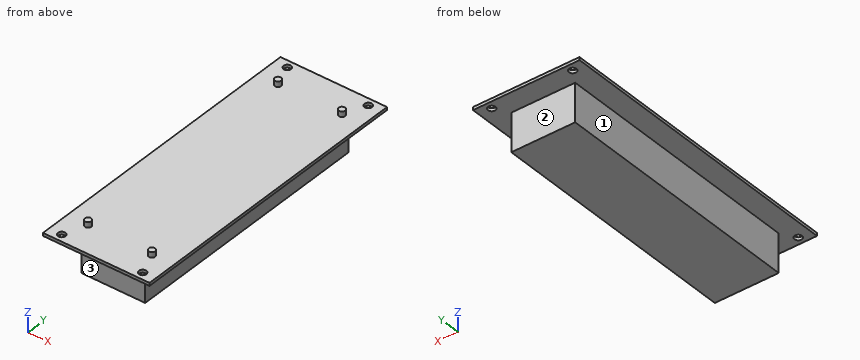
from build123d import *

# Parameters (mm, degrees)
SKETCH1_W           = 50
SKETCH1_H           = 140
BOSS_EXTRUDE1_DEPTH = 0.7
SKETCH3_W           = 30
SKETCH3_H           = 120
BOSS_EXTRUDE2_DEPTH = 18
SKETCH4_R           = 1.75
CUT_EXTRUDE1_DEPTH  = 1.4
SKETCH5_R           = 1.5
BOSS_EXTRUDE3_DEPTH = 2.5


with BuildPart() as part:
    # Sketch1 → Boss-Extrude1 (new, symmetric)
    with BuildSketch(Plane.XY):
        Rectangle(SKETCH1_W, SKETCH1_H)
    extrude(amount=BOSS_EXTRUDE1_DEPTH, both=True)

    # Sketch3 → Boss-Extrude2 (add)
    with BuildSketch(Plane(origin=(0, 0, -0.7), x_dir=(-1, 0, 0), z_dir=(0, 0, -1))):
        Rectangle(SKETCH3_W, SKETCH3_H)
    extrude(amount=BOSS_EXTRUDE2_DEPTH)

    # Sketch4 → Cut-Extrude1 (cut)
    with BuildSketch(Plane(origin=(0, 0, -0.7), x_dir=(-1, 0, 0), z_dir=(0, 0, -1))):
        with Locations((-19, 66.5)):
            Circle(SKETCH4_R)
        with Locations((19, 66.5)):
            Circle(SKETCH4_R)
        with Locations((-19, -66.5)):
            Circle(SKETCH4_R)
        with Locations((19, -66.5)):
            Circle(SKETCH4_R)
    extrude(amount=-CUT_EXTRUDE1_DEPTH, mode=Mode.SUBTRACT)

    # Sketch5 → Boss-Extrude3 (add)
    with BuildSketch(Plane.XY.offset(0.7)):
        with Locations(Location((15, 56, 0), (0, 0, 180))):
            Circle(SKETCH5_R)
        with Locations(Location((-15, 56, 0), (0, 0, 180))):
            Circle(SKETCH5_R)
        with Locations(Location((-15, -56, 0), (0, 0, 180))):
            Circle(SKETCH5_R)
        with Locations(Location((15, -56, 0), (0, 0, 180))):
            Circle(SKETCH5_R)
    extrude(amount=BOSS_EXTRUDE3_DEPTH)


solid = part.part
Source: CAD feature listing. Evaluate the final solid. Frame: model axes, mm. Face numbers are marked on the shaded views. A direction names the side the tool comes from. Round coordinates to 2 decimals unless told otherwise and drop trailing zeros. Loops run counter-clockwise (first coordinate to the right, second up) from the corner with the lowest first, then second, coordinate; pieces in that order, holes last.
Q1. Access query for the marked faces 1, 2 and 3. Directions: +Z, -Z, +X, -X, +Y, -Y. A direction counts if a zero-diameter tool reaches every point of the face in a straight line with its end or side. Return the directions, or none.
Q2. First-contact query: P1, Ø8, axis at y = 24.5, z = -10, coming from the +X side; P2, Ø1.5, axis at x = -10.5, y = 0, coming from the +Z side; P3, Ø9, axis at y = -21.5, z = -7, coming from the -X side. Flat tips, straight axial feed; report the tip coordinate or a pass-through.
Q3. Ray query, line 1 (Y direction, x = -19, z = 0.2); line 2 (X direction, y = 66.5, z = 0); line 3 (Z direction, x = 0.5, y = -30). Return the intervals inside material, ascending.
Q4. Section A-A, the plane x = 19. Return loops of the section in (y, z), plus the area to 3 significant figures.
Q5. Section D-D, the plane x = 10.5. Return loops of the section in (y, z), plus the area to 3 significant figures.
Q6. Section B-B, the plane y = 66.5. Return loops of the section in (x, z).
Q7. Section C-C, the plane y = -44.5. Return loops of the section in (x, z), plus the area to 3 significant figures.
Solutions:
1. face 1: -Z, -X, +Y, -Y
1. face 2: -Z, +X, -X, +Y
1. face 3: -Z, +X, -X, -Y
2. P1: stops at x = 15
2. P2: stops at z = 0.7
2. P3: stops at x = -15
3. line 1: y = -70 to -68.25, -64.75 to 64.75, 68.25 to 70
3. line 2: x = -25 to -20.75, -17.25 to 17.25, 20.75 to 25
3. line 3: z = -18.7 to 0.7
4. outline: (-70, -0.7) - (-68.25, -0.7) - (-68.25, 0.7) - (-70, 0.7) - close; (-64.75, -0.7) - (64.75, -0.7) - (64.75, 0.7) - (-64.75, 0.7) - close; (68.25, -0.7) - (70, -0.7) - (70, 0.7) - (68.25, 0.7) - close
4. area: 186 mm2
5. outline: (-70, -0.7) - (-60, -0.7) - (-60, -18.7) - (60, -18.7) - (60, -0.7) - (70, -0.7) - (70, 0.7) - (-70, 0.7) - close
5. area: 2,360 mm2
6. outline: (-25, -0.7) - (-20.75, -0.7) - (-20.75, 0.7) - (-25, 0.7) - close; (-17.25, -0.7) - (17.25, -0.7) - (17.25, 0.7) - (-17.25, 0.7) - close; (20.75, -0.7) - (25, -0.7) - (25, 0.7) - (20.75, 0.7) - close
7. outline: (-25, -0.7) - (-15, -0.7) - (-15, -18.7) - (15, -18.7) - (15, -0.7) - (25, -0.7) - (25, 0.7) - (-25, 0.7) - close
7. area: 610 mm2
